Geometry: see drawing. Coordinates: mm, zero at the bounding-box minimum. A direction names the side the tool comes from. Give positions to 0.01 mm unless a question says otherwise; leave off trailing zeros. Order: outer loops, then holes, each group sorted by start corner. A loop starts at its lowest first (then second) coordinate and runs counter-clockwise, first axis right, second up. Notation, with made-up numbers: (67, 3) - (105, 3) arc R13 cw to (105, 8) - close; hole circle Ø7 at (11.5, 88). An arc over 180 degrees is marked (long way). Write each question's results on one line, items separated by ' | '. Start each with the question number.
Item 1: Contact query for flat-ended pins moving along their axis: pin 1 Ø2.5 at (y, z) = (5, 27) entering from -X; pin 2 Ø2 at (y, z) = (6.5, 20) entering from +X (1 decimal); pin 3 Ø1 at (y, z) = (9.5, 36) entering from +X; pin 4 Ø5 at (x, y) = (26, 11) entering from +Z. Output: stop coordinate, or through.
Item 2: Section A-A on z = 28.5. Output: boundary loops of the cut face in (x, y) (1 decimal).
Item 3: Section D-D on x = 31.5. Output: boundary loops of the cut face in (y, z).
Item 4: Section B-B on y = 1.5. Output: boundary loops of the cut face in (x, z) (1 decimal).
Item 5: Line query: line 1 along Z through (x, y) = (11, 8.25); line 2 along X through (y, z) = (11.5, 25) (1 decimal); line 3 along Z through (x, y) = (15, 6.25) (1 decimal). Output: solid intervals per line, ascending.
Item 6: Mould query, pull axis Z, two halves, no side actions, for the marked faces 1, 2 and 3. Classes: released by +Z, released by -Z, zero draft, split by the parting line, or undercut.
Item 7: Set-up query: the marked faces 4 and 5. Return all of +Z, -Z, +X, -X, +Y, -Y with unobstructed straight access to the full face (end or side cutting, diameter ignored); none if empty.
Item 8: Section C-C on x = 26.5. Output: boundary loops of the cut face in (y, z), and give its area (3 significant figures).
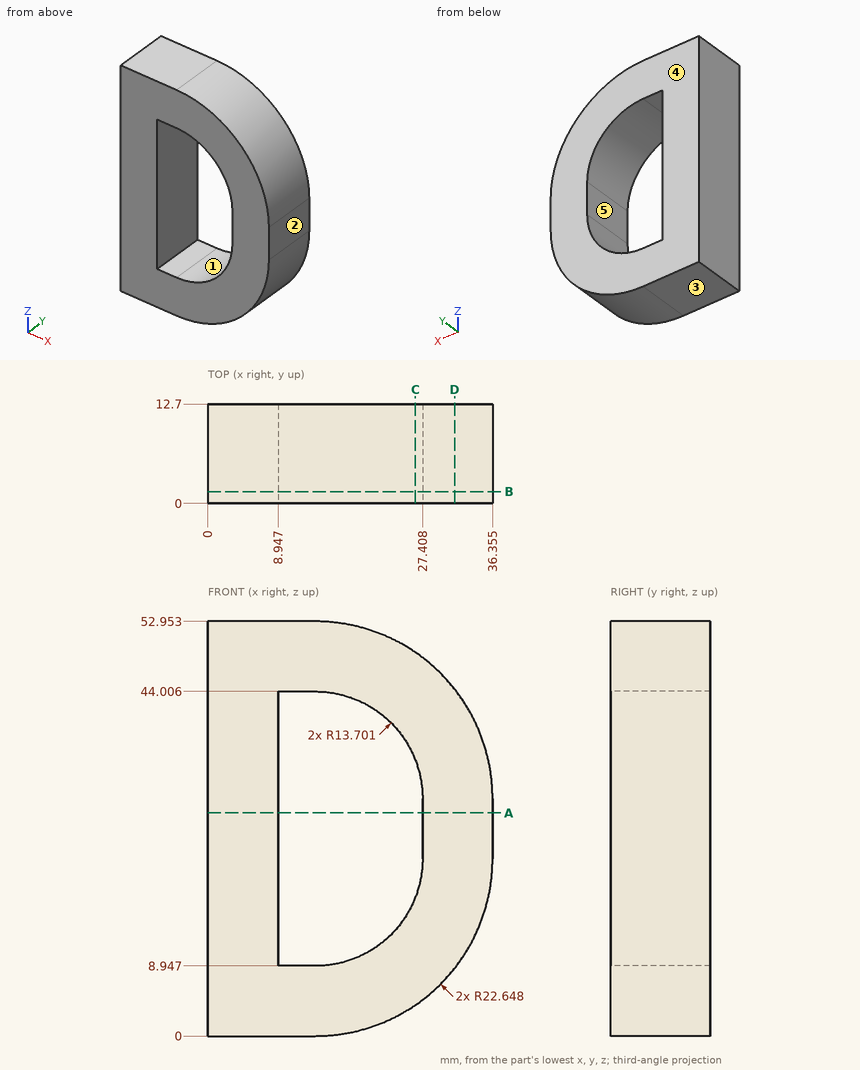
Evaluation:
1) pin 1: stops at x = 0 | pin 2: stops at x = 36.3 | pin 3: stops at x = 35.75 | pin 4: stops at z = 50.73
2) outline: (0, 0) - (8.9, 0) - (8.9, 12.7) - (0, 12.7) - close; (27.4, 0) - (36.4, 0) - (36.4, 12.7) - (27.4, 12.7) - close
3) outline: (0, 8.64) - (12.7, 8.64) - (12.7, 44.32) - (0, 44.32) - close
4) outline: (0, 0) - (13.7, 0) arc R22.6 ccw to (36.4, 22.6) - (36.4, 30.3) arc R22.6 ccw to (13.7, 53) - (0, 53) - close; hole (8.9, 8.9) - (13.7, 8.9) arc R13.7 ccw to (27.4, 22.6) - (27.4, 30.3) arc R13.7 ccw to (13.7, 44) - (8.9, 44) - close
5) line 1: z = 0 to 8.95, 44.01 to 52.95 | line 2: x = 0 to 8.9, 27.4 to 36.4 | line 3: z = 0 to 9, 43.9 to 52.9
6) face 1: undercut | face 2: zero draft | face 3: released by -Z
7) face 4: +Z, -Z, +X, -X, +Y | face 5: +Y, -Y
8) outline: (0, 3.96) - (12.7, 3.96) - (12.7, 17.74) - (0, 17.74) - close; (0, 35.21) - (12.7, 35.21) - (12.7, 48.99) - (0, 48.99) - close | area: 350 mm^2
